Here's how the part is built. I have some questions about the finished solid (model axes, mm). Round coordinates to 2 decimals unless told otherwise and drop trailing zeros. Loops run counter-clockwise (first coordinate to the right, second up) from the corner with the lowest first, then second, coordinate; pieces in that order, holes last. Notation, with made-up numbers: (58.25, -15.5) -> (111.25, -15.5) arc R30 cw to (111.25, 20.5) -> close; hole circle Ø4 at (4.25, 26.25). An arc over 180 degrees is marked (long way). One line per item, written item: value. Start each with the question number.
```python
from build123d import *

# Parameters (mm, degrees)
F0_W          = 50
F0_H          = 50
F1_DEPTH      = 50
F4_DEPTH      = 50
F5_DEPTH      = 51
F6_T          = -2.5
F8_ANGLE_BACK = 89.955
F8_ANGLE      = 179.91
F10_DEPTH     = 2
F12_DEPTH     = 13


with BuildPart() as f1:
    # F0 (on Top) → F1 (new body)
    with BuildSketch(Plane.XY):
        Rectangle(F0_W, F0_H)
    extrude(amount=F1_DEPTH)

    # F3 (on face) → F4 (cut, through all)
    with BuildSketch(Plane.YZ.offset(25)):
        Polygon((-25, 1.3375796843), (-25, 0), (0, 50), (-25, 50), align=None)
        Polygon((25, 50), (0, 50), (25, 0), align=None)
    extrude(amount=-F4_DEPTH, mode=Mode.SUBTRACT)

    # F2 (on face) → F5 (cut, up to face)
    with BuildSketch(Plane.XZ.offset(25)):
        Polygon((-25, 50), (-25, 0), (0, 50), align=None)
        Polygon((25, 50), (0, 50), (25, 0), align=None)
    extrude(amount=-F5_DEPTH, mode=Mode.SUBTRACT)

    # F6
    f6_openings = [f1.faces().sort_by_distance(p)[0] for p in [
        (0, 0, 0),
    ]]
    offset(amount=F6_T, openings=f6_openings)

    # F7 (on Front) → F8 (revolve)
    with BuildSketch(Plane.XZ, mode=Mode.PRIVATE) as f8_sk:
        Polygon((-7.5, 50), (-7.5, 35), (0, 50), align=None)
        Polygon((7.5, 50), (0, 50), (7.5, 35), align=None)
    revolve(f8_sk.sketch.rotate(Axis((0, 0, 42.5), (0, 0, -1)), -F8_ANGLE_BACK), axis=Axis((0, 0, 42.5), (0, 0, -1)), revolution_arc=F8_ANGLE)

    # F9 (on face) → F10 (join)
    with BuildSketch(Plane.XY.offset(50)):
        with BuildLine():
            Line((0, 0), (0.0058904856, 7.4999976868))
            ThreePointArc((0.0058904856, 7.4999976868), (0, 7.5), (-0.0058904856, 7.4999976868))
            Line((-0.0058904856, 7.4999976868), (0, 0))
        make_face()
        with BuildLine():
            ThreePointArc((-5.3033008589, 5.3033008589), (-2.8701257427, -6.9290964938), (7.5, 0))
            ThreePointArc((7.5, 0), (6.9290964938, 2.8701257427), (5.3033008589, 5.3033008589))
            ThreePointArc((5.3033008589, 5.3033008589), (2.8728465712, 6.9279688638), (0.0058904856, 7.4999976868))
            Line((0.0058904856, 7.4999976868), (0, 0))
            Line((0, 0), (-0.0058904856, 7.4999976868))
            ThreePointArc((-0.0058904856, 7.4999976868), (-2.8728465712, 6.9279688638), (-5.3033008589, 5.3033008589))
        make_face()
    extrude(amount=-F10_DEPTH)

    # F11 (on face) → F12 (join)
    with BuildSketch(Plane.XY.offset(50)):
        with BuildLine():
            ThreePointArc((-0.0047123885, 5.9999981494), (0, 6), (0.0047123885, 5.9999981494))
            Line((0.0047123885, 5.9999981494), (0.0058904856, 7.4999976868))
            ThreePointArc((0.0058904856, 7.4999976868), (0, 7.5), (-0.0058904856, 7.4999976868))
            Line((-0.0058904856, 7.4999976868), (-0.0047123885, 5.9999981494))
        make_face()
        with BuildLine():
            ThreePointArc((-0.0047123885, -5.9999981494), (-6, 0), (-0.0047123885, 5.9999981494))
            Line((-0.0047123885, 5.9999981494), (-0.0058904856, 7.4999976868))
            ThreePointArc((-0.0058904856, 7.4999976868), (-7.5, 0), (-0.0058904856, -7.4999976868))
            Line((-0.0058904856, -7.4999976868), (-0.0047123885, -5.9999981494))
        make_face()
        with BuildLine():
            Line((0.0058904856, -7.4999976868), (0.0047123885, -5.9999981494))
            ThreePointArc((0.0047123885, -5.9999981494), (0, -6), (-0.0047123885, -5.9999981494))
            Line((-0.0047123885, -5.9999981494), (-0.0058904856, -7.4999976868))
            ThreePointArc((-0.0058904856, -7.4999976868), (0, -7.5), (0.0058904856, -7.4999976868))
        make_face()
        with BuildLine():
            ThreePointArc((0.0047123885, 5.9999981494), (4.244306441, 4.2409742789), (6, 0))
            ThreePointArc((6, 0), (4.244306441, -4.2409742789), (0.0047123885, -5.9999981494))
            Line((0.0047123885, -5.9999981494), (0.0058904856, -7.4999976868))
            ThreePointArc((0.0058904856, -7.4999976868), (5.3053830513, -5.3012178487), (7.5, 0))
            ThreePointArc((7.5, 0), (5.3053830513, 5.3012178487), (0.0058904856, 7.4999976868))
            Line((0.0058904856, 7.4999976868), (0.0047123885, 5.9999981494))
        make_face()
    extrude(amount=-F12_DEPTH)


solid = f1.part
```
Q1. I want a section at D-D on z = 31.5. Please give me the cut outline in (x, y), plus the area to 3 significant figures.
Q2. I want a section at B-B on x = 2.5. Please give me the cut outline in (y, z).
Q3. If I drill on line 1 along X through (y, z) = (10, 22.5); line 2 along Y through (x, z) = (7, 23); line 3 along X through (y, z) = (0.5, 17), over which ranges is the centre line in solid material (lowest first)?
Q4. I want a section at A-A on z = 23. Please give me the cut outline in (x, y).
Q5. I want a section at C-C on y = 18. Please give me the cut outline in (x, z), plus the area to 3 significant figures.
Q6. If we mould it in two halves opening along Y, with no side actions, what happens to faces 1 (the flat face through (0, 0, 50)), 2 (the flat face through (13.414, -0.311, 17.581)), 3 (the flat face through (0.3, -17.5, 15))? For each: released by +Y, released by -Y, zero draft, split by the parting line, or undercut.
Q7. Will these pins go through, and if not, where does the flat tip stop? P1, Ø12, axis at x = 20, y = 8.5, coming from the +Z side; P2, Ø12, axis at x = -19, y = 5, coming from the +Z side; P3, Ø3, axis at y = -11.5, z = 21.5, coming from the -X side; P4, Ø1.5, axis at y = -16.5, z = 22.5, coming from the -X side.
Answers below:
1. outline: (-9.25, -9.25) -> (9.25, -9.25) -> (9.25, 9.25) -> (-9.25, 9.25) -> close; hole (-6.45, -6.45) -> (6.45, -6.45) -> (6.45, 6.45) -> (-6.45, 6.45) -> close
1. area: 176 mm^2
2. outline: (-25, 0) -> (-22.2, 0) -> (-2.5, 39.41) -> (2.5, 39.41) -> (22.2, 0) -> (25, 0) -> (7.07, 35.86) -> (7.07, 50) -> (-7.07, 50) -> (-7.07, 35.86) -> close
3. line 1: x = -13.75 to -10.95, 10.95 to 13.75
3. line 2: y = -13.5 to -10.7, 10.7 to 13.5
3. line 3: x = -16.5 to -13.7, 13.7 to 16.5
4. outline: (-13.5, -13.5) -> (13.5, -13.5) -> (13.5, 13.5) -> (-13.5, 13.5) -> close; hole (-10.7, -10.7) -> (10.7, -10.7) -> (10.7, 10.7) -> (-10.7, 10.7) -> close
5. outline: (-25, 0) -> (-22.2, 0) -> (-18, 8.41) -> (18, 8.41) -> (22.2, 0) -> (25, 0) -> (18, 14) -> (-18, 14) -> close
5. area: 264 mm^2
6. face 1: zero draft
6. face 2: undercut
6. face 3: released by -Y
7. P1: stops at z = 22
7. P2: stops at z = 24
7. P3: stops at x = -15
7. P4: passes through
